The model under review builds one solid part; all positions refer to its coordinate system, in mm. A direction names the side the tool comes from. Coordinates: 2 decimals unless noted, no trailing zeros. Write each loop counter-clockwise with the first axis right and the second up, starting at its lowest first coordinate (ties: lowest second). Pieces come first, ordered by that corner, then holes. Notation, with made-up numbers: (72, -2) - (125, -2) arc R29 ccw to (125, 35) - close; hole circle Ø2 at (56.5, -35). An arc over 180 degrees is marked (long way). Answer as CSV lines item,"result". Start each with the question number.
```python
from build123d import *

# Parameters (mm, degrees)
SKETCH_1_R               = 1.5
EXTRUDE_1_DEPTH          = 2.3
SKETCH_2_R               = 4.4
EXTRUDE_2_DEPTH          = 3.2
SKETCH_3_R               = 4.4
SKETCH_3_R_2             = 3.4
SKETCH_3_R_3             = 2.75
SKETCH_3_R_4             = 1.5
CUT_EXTRUDE_1_DEPTH      = 1
BOSS_EXTRUDE1_DEPTH      = 2
BOSS_EXTRUDE1_DEPTH_BACK = 2
SKETCH1_R                = 35
INTERSECT2_OUTLINE_R     = 4.4
INTERSECT2_OUTLINE_R_2   = 3.4
INTERSECT2_OUTLINE_R_3   = 2.75
INTERSECT2_DEPTH         = 5.5
INTERSECT2_START         = 1
INTERSECT2_2_OUTLINE_R   = 4.4
INTERSECT2_2_OUTLINE_R_2 = 3.4
INTERSECT2_2_OUTLINE_R_3 = 2.75
INTERSECT2_2_OUTLINE_R_4 = 1.5
INTERSECT2_2_DEPTH       = 4.5
FILLET1_R                = 10
SKETCH2_R                = 25
BOSS_EXTRUDE2_DEPTH      = 2
SKETCH3_R                = 27
BOSS_EXTRUDE3_DEPTH      = 2
SKETCH4_R                = 6
CUT_EXTRUDE1_DEPTH       = 2
CUT_EXTRUDE3_REACH       = 52.14
SKETCH5_R                = 2.5
CUT_EXTRUDE4_START       = -2
CUT_EXTRUDE4_DEPTH       = 2
CHAMFER1_SIZE            = 1


# Read off the part's stored shape, not the designer's step: Intersect2
with BuildPart() as part:
    # Эскиз1 → Бобышка-Вытянуть1 (new body)
    with BuildSketch(Plane.XY):
        with BuildLine():
            Line((-3.968626967, 4.5), (-16.888114198, 2.469689731))
            ThreePointArc((-16.888114198, 2.469689731), (-19, 0), (-16.888114198, -2.469689731))
            Line((-16.888114198, -2.469689731), (-3.968626967, -4.5))
            ThreePointArc((-3.968626967, -4.5), (0, -6), (3.968626967, -4.5))
            Line((3.968626967, -4.5), (16.888114198, -2.469689731))
            ThreePointArc((16.888114198, -2.469689731), (19, 0), (16.888114198, 2.469689731))
            Line((16.888114198, 2.469689731), (3.968626967, 4.5))
            ThreePointArc((3.968626967, 4.5), (0, 6), (-3.968626967, 4.5))
        make_face()
        Circle(SKETCH_1_R, mode=Mode.SUBTRACT)
    extrude(amount=EXTRUDE_1_DEPTH)

    # Эскиз2 → Бобышка-Вытянуть2 (add)
    with BuildSketch(Plane.XY.offset(2.3)):
        with Locations(Location((0, 0, 0), (0, 0, 180))):
            Circle(SKETCH_2_R)
        Polygon((0.333439775, 2.639447604), (0, 3.05), (-0.333439775, 2.639447604), (-0.758504156, 2.954178641), (-0.979368078, 2.473601404), (-1.469348706, 2.672735374), (-1.563759083, 2.15232973), (-2.087868673, 2.223354314), (-2.049893354, 1.695819264), (-2.575200173, 1.634271725), (-2.407225286, 1.132754236), (-2.900722375, 0.942501833), (-2.6133024, 0.498514094), (-3.043981522, 0.191511085), (-2.655176114, -0.167049522), (-2.995976115, -0.571513009), (-2.530215347, -0.822116802), (-2.75972251, -1.298626839), (-2.246271844, -1.42552746), (-2.35006539, -1.944143169), (-1.821186821, -1.939366985), (-1.792745019, -2.467501833), (-1.281669931, -2.33134895), (-1.122779886, -2.835818282), (-0.661621006, -2.576843686), (-0.382266362, -3.025949839), (0, -2.660425857), (0.382266362, -3.025949839), (0.661621006, -2.576843686), (1.122779886, -2.835818282), (1.281669931, -2.33134895), (1.792745019, -2.467501833), (1.821186821, -1.939366985), (2.35006539, -1.944143169), (2.246271844, -1.42552746), (2.75972251, -1.298626839), (2.530215347, -0.822116802), (2.995976115, -0.571513009), (2.655176114, -0.167049522), (3.043981522, 0.191511085), (2.6133024, 0.498514094), (2.900722375, 0.942501833), (2.407225286, 1.132754236), (2.575200173, 1.634271725), (2.049893354, 1.695819264), (2.087868673, 2.223354314), (1.563759083, 2.15232973), (1.469348706, 2.672735374), (0.979368078, 2.473601404), (0.758504156, 2.954178641), align=None, mode=Mode.SUBTRACT)
    extrude(amount=EXTRUDE_2_DEPTH)

    # Эскиз3 → Вырез-Вытянуть1 (cut)
    # profile 1 of 2: a face of its own
    with BuildSketch(Plane(origin=(0, 0, 0), x_dir=(-1, 0, 0), z_dir=(0, 0, -1))):
        Circle(SKETCH_3_R)
        Circle(SKETCH_3_R_2, mode=Mode.SUBTRACT)
    # profile 2 of 2: a face of its own
    with BuildSketch(Plane(origin=(0, 0, 0), x_dir=(-1, 0, 0), z_dir=(0, 0, -1))):
        Circle(SKETCH_3_R_3)
        Circle(SKETCH_3_R_4, mode=Mode.SUBTRACT)
    extrude(amount=-CUT_EXTRUDE_1_DEPTH, mode=Mode.SUBTRACT)


with BuildPart() as body_2:
    # Sketch1 → Boss-Extrude1 (new, two sides: drawn at the far end of the back side and taken through both)
    with BuildSketch(Plane(origin=(0, 0, 0), x_dir=(-1, 0, 0), z_dir=(0, 0, -1)).offset(-BOSS_EXTRUDE1_DEPTH_BACK)):
        Circle(SKETCH1_R)
    extrude(amount=BOSS_EXTRUDE1_DEPTH + BOSS_EXTRUDE1_DEPTH_BACK)


with BuildPart() as intersect2_tool:
    # Intersect2 outline → Intersect2 (new body)
    # profile 1 of 2: a face of its own
    with BuildSketch(Plane.XY):
        with BuildLine():
            ThreePointArc((3.968626967, 4.5), (0, 6), (-3.968626967, 4.5))
            Line((-3.968626967, 4.5), (-16.888114198, 2.469689731))
            ThreePointArc((-16.888114198, 2.469689731), (-19, 0), (-16.888114198, -2.469689731))
            Line((-16.888114198, -2.469689731), (-3.968626967, -4.5))
            ThreePointArc((-3.968626967, -4.5), (0, -6), (3.968626967, -4.5))
            Line((3.968626967, -4.5), (16.888114198, -2.469689731))
            ThreePointArc((16.888114198, -2.469689731), (19, 0), (16.888114198, 2.469689731))
            Line((16.888114198, 2.469689731), (3.968626967, 4.5))
        make_face()
        Circle(INTERSECT2_OUTLINE_R, mode=Mode.SUBTRACT)
    # profile 2 of 2: a face of its own
    with BuildSketch(Plane.XY):
        Circle(INTERSECT2_OUTLINE_R_2)
        Circle(INTERSECT2_OUTLINE_R_3, mode=Mode.SUBTRACT)
    extrude(amount=INTERSECT2_DEPTH)


with BuildPart() as part_1:
    add(part.part)

    # Intersect2: cut by intersect2_tool
    add(intersect2_tool.part, mode=Mode.SUBTRACT)


with BuildPart() as body_2_1:
    add(body_2.part)

    # Intersect2: cut by intersect2_tool
    add(intersect2_tool.part, mode=Mode.SUBTRACT)


with BuildPart() as intersect2_2_tool:
    # Intersect2 2 outline → Intersect2 2 (new body)
    # profile 1 of 2: a face of its own
    with BuildSketch(Plane.XY.offset(INTERSECT2_START)):
        Circle(INTERSECT2_2_OUTLINE_R)
        Circle(INTERSECT2_2_OUTLINE_R_2, mode=Mode.SUBTRACT)
    # profile 2 of 2: a face of its own
    with BuildSketch(Plane.XY.offset(INTERSECT2_START)):
        Circle(INTERSECT2_2_OUTLINE_R_3)
        Circle(INTERSECT2_2_OUTLINE_R_4, mode=Mode.SUBTRACT)
    extrude(amount=INTERSECT2_2_DEPTH)


with BuildPart() as part_2:
    add(part_1.part)

    # Intersect2 2: cut by intersect2_2_tool
    add(intersect2_2_tool.part, mode=Mode.SUBTRACT)


with BuildPart() as body_2_2:
    add(body_2_1.part)

    # Intersect2 2: cut by intersect2_2_tool
    add(intersect2_2_tool.part, mode=Mode.SUBTRACT)

    # Fillet1
    # the kernel refuses this fillet: 10 mm, written as the material it takes off along each edge
    with BuildSketch(Plane(origin=(0, 0, 2), x_dir=(-1, 0, 0), z_dir=(0, -1, 0))) as fillet1_piece_1:
        with BuildLine():
            CenterArc((27, 10), FILLET1_R, 270, 53.130102354)
            Line((27, 0), (27, -0.2))
            Line((27, -0.2), (35, -0.2))
            Line((35, -0.2), (35.2, 0))
            ThreePointArc((35.2, 0), (35.2, 2), (35.16, 3.88))
            Line((35.16, 3.88), (35, 4))
        make_face()
    revolve(axis=Axis((0, 0, 2), (0, 0, -1)), mode=Mode.SUBTRACT)


with BuildPart() as body_2_2_1:
    # Mirror9: mirrored copy
    add(body_2_2.part.mirror(Plane.XY.offset(-3)))


with BuildPart() as body_2_3:
    add(body_2_2.part)

    add(body_2_2_1.part)  # Boss-Extrude2 merges body 2 2
    # Sketch2 → Boss-Extrude2 (add)
    with BuildSketch(Plane(origin=(0, 0, -2), x_dir=(-1, 0, 0), z_dir=(0, 0, -1))):
        Circle(SKETCH2_R)
    extrude(amount=BOSS_EXTRUDE2_DEPTH)

    # Sketch3 → Boss-Extrude3 (add)
    with BuildSketch(Plane(origin=(0, 0, -8), x_dir=(-1, 0, 0), z_dir=(0, 0, -1))):
        Circle(SKETCH3_R)
    extrude(amount=-BOSS_EXTRUDE3_DEPTH)

    # Sketch4 → Cut-Extrude1 (cut)
    with BuildSketch(Plane.XY):
        Circle(SKETCH4_R)
    extrude(amount=CUT_EXTRUDE1_DEPTH, mode=Mode.SUBTRACT)

    # Sketch5 → Cut-Extrude3 (cut, up to next)
    with BuildSketch(Plane.XY, mode=Mode.PRIVATE) as cut_extrude3_sk1:
        Circle(SKETCH5_R)
    cut_extrude3_tool1 = extrude(cut_extrude3_sk1.sketch, amount=-CUT_EXTRUDE3_REACH, mode=Mode.PRIVATE) & body_2_3.part
    add(cut_extrude3_tool1.solids().sort_by_distance((0, 0, 0))[0], mode=Mode.SUBTRACT)

    # Sketch6 → Cut-Extrude4 (cut)
    with BuildSketch(Plane.XY.offset(2).offset(CUT_EXTRUDE4_START)):
        with BuildLine():
            Line((16.919163334, 2.66726491), (4.056712891, 4.68861179))
            ThreePointArc((4.056712891, 4.68861179), (0, 6.2), (-4.056712891, 4.68861179))
            Line((-4.056712891, 4.68861179), (-16.919163334, 2.66726491))
            ThreePointArc((-16.919163334, 2.66726491), (-19.2, 0), (-16.919163334, -2.66726491))
            Line((-16.919163334, -2.66726491), (-4.056712891, -4.68861179))
            ThreePointArc((-4.056712891, -4.68861179), (0, -6.2), (4.056712891, -4.68861179))
            Line((4.056712891, -4.68861179), (16.919163334, -2.66726491))
            ThreePointArc((16.919163334, -2.66726491), (19.2, 0), (16.919163334, 2.66726491))
        make_face()
    extrude(amount=CUT_EXTRUDE4_DEPTH, mode=Mode.SUBTRACT)

    # Chamfer1
    chamfer1_edges = [body_2_3.edges().sort_by_distance(p)[0] for p in [
        (0, 6.2, 2),
        (-10.487938112, 3.67793835, 2),
        (-19.2, 0, 2),
        (-10.487938112, -3.67793835, 2),
        (0, -6.2, 2),
        (10.487938112, -3.67793835, 2),
        (19.2, 0, 2),
        (10.487938112, 3.67793835, 2),
    ]]
    chamfer(chamfer1_edges, length=CHAMFER1_SIZE)


solid = body_2_3.part
```
(1) Add section B-B on y = 0. Give the boundary of the cut face in (x, z).
(2) For pin 1 (2 mm diameter, centred on x = -24.5, z = 0.5, fed in from -Y); pin 2 (6 mm diameter, centred on y = 19.5, z = 0, fed in from -X); pin 3 (13.5 mm diameter, centred on x = -6.5, y = 3, fed in from +Z); pin 4 (3 mm diameter, centred on y = 1, z = 0.5, fed in from -X), all flat-tipped, find the tip position at first contact; note any pin that passes through.
(3) Wall thickness on line 1 (Z direction, x = 5, y = 3.5); line 2 (X direction, y = 1.5, z = -6.5); line 3 (Z direction, x = -23, y = -19): over which ranges is each line inside the solid? List them lowest first.
(4) Add section A-A on x = 0. Give the boundary of the cut face in (y, z), then the cut area to 3 significant figures.
(5) The part is to be moulded in two halves that separate along X. For faces 1 (the flat face through (24, 8, -4)), 2 (the cylindrical face through (-23.846, 7.509, -2.986)), 3 (the cylindrical face through (-0.54, -2.44, -3.94)), say which applies: released by +X, released by -X, zero draft, split by the parting line, or undercut.
(6) For faces 4 (the flat face through (24, 8, -2)), 5 (the flat face through (-6, 0, -8)), 6 (the flat face through (10.657, 4.165, 1.507)), list the 3-axis set-ups (+Z, -Z, +X, -X, +Y, -Y) from which the entire face can be reached by the end or side of a thin tool; tool diameter is ignored.
(7) Add section C-C on z = -5.75. Give the boundary of the cut face in (x, y), then the cut area to 3 significant figures.
Reported:
1,outline,"(-35, -4) arc R10 ccw to (-27, -8) - (-2.5, -8) - (-2.5, 0) - (-19.2, 0) - (-19.2, 1) - (-20.2, 2) - (-27, 2) arc R10 ccw to (-35, -2) - (-25, -2) - (-25, -4) - close; (2.5, -8) - (27, -8) arc R10 ccw to (35, -4) - (25, -4) - (25, -2) - (35, -2) arc R10 ccw to (27, 2) - (20.2, 2) - (19.2, 1) - (19.2, 0) - (2.5, 0) - close"
2,pin 1,"y = -23.31"
2,pin 2,"x = -30.45"
2,pin 3,"z = 2"
2,pin 4,"x = -34.13"
3,line 1,"-8 to 0"
3,line 2,"-32.23 to -2, 2 to 32.23"
3,line 3,"-7.59 to -4, -2 to 1.59"
4,outline,"(-35, -4) arc R10 ccw to (-27, -8) - (-2.5, -8) - (-2.5, 0) - (-6.2, 0) - (-6.2, 1) - (-7.2, 2) - (-27, 2) arc R10 ccw to (-35, -2) - (-25, -2) - (-25, -4) - close; (2.5, -8) - (27, -8) arc R10 ccw to (35, -4) - (25, -4) - (25, -2) - (35, -2) arc R10 ccw to (27, 2) - (7.2, 2) - (6.2, 1) - (6.2, 0) - (2.5, 0) - close"
4,area,"556 mm²"
5,face 1,"zero draft"
5,face 2,"split by the parting line"
5,face 3,"undercut"
6,face 4,"none"
6,face 5,"-Z, +X, -X, +Y, -Y"
6,face 6,"+Z"
7,outline,"circle Ø66.64 at (0, 0); hole circle Ø5 at (0, 0)"
7,area,"3,470 mm²"
